Could you check a few things on this model? Use its own coordinates, in mm. Face numbers are marked on the shaded views. A direction names the side the tool comes from. Give positions to 0.01 mm unless a question says otherwise; leave off trailing zeros. Loops run counter-clockwise (first coordinate to the right, second up) from the corner with the lowest first, then second, coordinate; pieces in that order, holes last. Notation, with made-up numbers: M 28.25,60.5 L 63.25,60.5 A28 ccw 63.25,78.5 Z; hole C 39.25,-36 d9. An arc over 180 degrees is marked long. Answer in a Markdown table with one row per item. Add a question column.
1. Which directions (+Z, -Z, +X, -X, +Y, -Y) give clear straight access to the entire face, cutting with the end or side of a thin tool? Please do the marked faces 1 and 2.
2. If we section it at A-A on x = 12: List the corners of the cut face in (y, z) for me, then the cut area to 3 significant figures.
3. Thinking about a two-plate mould opening in Y: for the marked faces 3, 4 and 5, which applies, released by +Y, released by -Y, zero draft, split by the parting line, or undercut?
4. If we section it at B-B on z = 2.8: List the corners of the cut face in (x, y) for me.
5. If we section it at D-D on z = 1.05: List the corners of the cut face in (x, y) for me, then the cut area to 3 significant figures.
6. If we section it at C-C on y = 4.5: List the corners of the cut face in (x, z) for me.
7. I need wall thicknesses on line 1 along Y through (x, z) = (14.5, 2.5); line 2 along Y through (x, z) = (-10.5, 0.2); line 3 along Z through (x, y) = (5, 1.75). Which ranges of each line are inside material? Lowest first, please. Write a range as from..to.
8. I'm going to push flat-ended pins straight in: pin 1 Ø0.9 at (x, z) = (7.5, 4) entering from +Y; pin 2 Ø1.5 at (x, z) = (12.5, 4) entering from -Y; pin 3 Ø2 at (y, z) = (3, 4) entering from -X; pin 4 Ø2.5 at (x, z) = (11, 2.5) entering from +Y. Where does each tip first touch, or does it pass through?
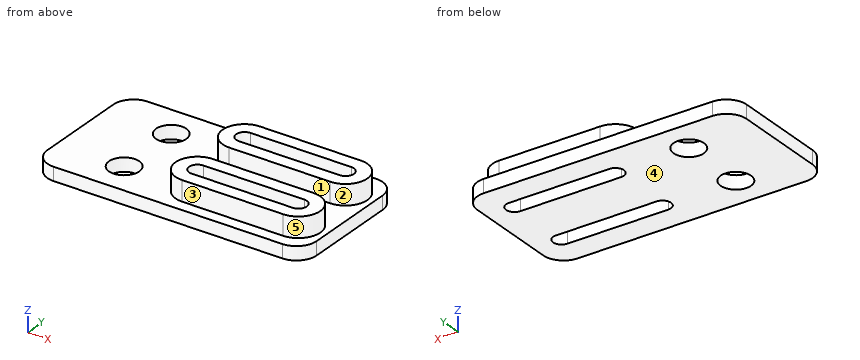
```python
from build123d import *

# Parameters (mm, degrees)
SZKIC1_W                    = 40
SZKIC1_H                    = 20
SZKIC1_R                    = 2.25
DODANIE_WYCI_GNI_CIE1_DEPTH = 2
DODANIE_WYCI_GNI_CIE2_DEPTH = 5
ZAOKR_GLENIE1_R             = 3


with BuildPart() as part:
    # Szkic1 → Dodanie-wyci_gni_cie1 (new body)
    with BuildSketch(Plane.XY):
        with Locations((0.494567618, 0.286392586)):
            Rectangle(SZKIC1_W, SZKIC1_H)
        with Locations((-9.505432382, -4.713607414)):
            Circle(SZKIC1_R, mode=Mode.SUBTRACT)
        with Locations((-9.505432382, 5.286392586)):
            Circle(SZKIC1_R, mode=Mode.SUBTRACT)
        with BuildLine():
            ThreePointArc((16.387577827, 2.036392586), (19.637577827, 5.286392586), (16.387577827, 8.536392586))
            Line((16.387577827, 8.536392586), (1.387577827, 8.536392586))
            ThreePointArc((1.387577827, 8.536392586), (-1.862422173, 5.286392586), (1.387577827, 2.036392586))
            Line((1.387577827, 2.036392586), (16.387577827, 2.036392586))
        make_face(mode=Mode.SUBTRACT)
        with BuildLine():
            ThreePointArc((16.387577827, -7.963607414), (19.637577827, -4.713607414), (16.387577827, -1.463607414))
            Line((16.387577827, -1.463607414), (1.387577827, -1.463607414))
            ThreePointArc((1.387577827, -1.463607414), (-1.862422173, -4.713607414), (1.387577827, -7.963607414))
            Line((1.387577827, -7.963607414), (16.387577827, -7.963607414))
        make_face(mode=Mode.SUBTRACT)
    extrude(amount=DODANIE_WYCI_GNI_CIE1_DEPTH)

    # Szkic1_3 → Dodanie-wyci_gni_cie2 (add)
    # profile 1 of 2: a face of its own
    with BuildSketch(Plane.XY):
        with BuildLine():
            Line((1.387577827, -1.463607414), (16.387577827, -1.463607414))
            ThreePointArc((16.387577827, -1.463607414), (19.637577827, -4.713607414), (16.387577827, -7.963607414))
            Line((16.387577827, -7.963607414), (1.387577827, -7.963607414))
            ThreePointArc((1.387577827, -7.963607414), (-1.862422173, -4.713607414), (1.387577827, -1.463607414))
        make_face()
        with BuildLine():
            Line((1.387577827, -3.463607414), (16.387577827, -3.463607414))
            ThreePointArc((16.387577827, -3.463607414), (17.637577827, -4.713607414), (16.387577827, -5.963607414))
            Line((16.387577827, -5.963607414), (1.387577827, -5.963607414))
            ThreePointArc((1.387577827, -5.963607414), (0.137577827, -4.713607414), (1.387577827, -3.463607414))
        make_face(mode=Mode.SUBTRACT)
    # profile 2 of 2: a face of its own
    with BuildSketch(Plane.XY):
        with BuildLine():
            Line((1.387577827, 8.536392586), (16.387577827, 8.536392586))
            ThreePointArc((16.387577827, 8.536392586), (19.637577827, 5.286392586), (16.387577827, 2.036392586))
            Line((16.387577827, 2.036392586), (1.387577827, 2.036392586))
            ThreePointArc((1.387577827, 2.036392586), (-1.862422173, 5.286392586), (1.387577827, 8.536392586))
        make_face()
        with BuildLine():
            Line((1.387577827, 6.536392586), (16.387577827, 6.536392586))
            ThreePointArc((16.387577827, 6.536392586), (17.637577827, 5.286392586), (16.387577827, 4.036392586))
            Line((16.387577827, 4.036392586), (1.387577827, 4.036392586))
            ThreePointArc((1.387577827, 4.036392586), (0.137577827, 5.286392586), (1.387577827, 6.536392586))
        make_face(mode=Mode.SUBTRACT)
    extrude(amount=DODANIE_WYCI_GNI_CIE2_DEPTH)

    # Zaokr_glenie1
    zaokr_glenie1_edges = [part.edges().sort_by_distance(p)[0] for p in [
        (20.494567618, -9.713607414, 1),
        (-19.505432382, -9.713607414, 1),
        (-19.505432382, 10.286392586, 1),
        (20.494567618, 10.286392586, 1),
    ]]
    fillet(zaokr_glenie1_edges, radius=ZAOKR_GLENIE1_R)


solid = part.part
```
Results:
| question | item | result |
|---|---|---|
| 1 | face 1 | +Z, +X, -X |
| 1 | face 2 | +Z, +X |
| 2 | outline | M -9.71,0 L -5.96,0 L -5.96,5 L -7.96,5 L -7.96,2 L -9.71,2 Z; M -3.46,0 L 4.04,0 L 4.04,5 L 2.04,5 L 2.04,2 L -1.46,2 L -1.46,5 L -3.46,5 Z; M 6.54,0 L 10.29,0 L 10.29,2 L 8.54,2 L 8.54,5 L 6.54,5 Z |
| 2 | area | 54.0 mm2 |
| 3 | face 3 | released by -Y |
| 3 | face 4 | zero draft |
| 3 | face 5 | undercut |
| 4 | outline | M 1.39,-7.96 L 16.39,-7.96 A3.25 ccw 16.39,-1.46 L 1.39,-1.46 A3.25 ccw Z; M 1.39,2.04 L 16.39,2.04 A3.25 ccw 16.39,8.54 L 1.39,8.54 A3.25 ccw Z; hole M 1.39,-5.96 L 16.39,-5.96 A1.25 ccw 16.39,-3.46 L 1.39,-3.46 A1.25 ccw Z; hole M 1.39,4.04 L 16.39,4.04 A1.25 ccw 16.39,6.54 L 1.39,6.54 A1.25 ccw Z |
| 5 | outline | M -19.51,-6.71 A3 ccw -16.51,-9.71 L 17.49,-9.71 A3 ccw 20.49,-6.71 L 20.49,7.29 A3 ccw 17.49,10.29 L -16.51,10.29 A3 ccw -19.51,7.29 Z; hole C -9.51,-4.71 d4.5; hole C -9.51,5.29 d4.5; hole M 1.39,-5.96 L 16.39,-5.96 A1.25 ccw 16.39,-3.46 L 1.39,-3.46 A1.25 ccw Z; hole M 1.39,4.04 L 16.39,4.04 A1.25 ccw 16.39,6.54 L 1.39,6.54 A1.25 ccw Z |
| 5 | area | 676 mm2 |
| 6 | outline | M -19.51,0 L -11.61,0 L -11.61,2 L -19.51,2 Z; M -7.4,0 L 0.42,0 L 0.42,5 L -1.77,5 L -1.77,2 L -7.4,2 Z; M 17.36,0 L 20.49,0 L 20.49,2 L 19.54,2 L 19.54,5 L 17.36,5 Z |
| 7 | line 1 | -7.96..-5.96, -3.46..-1.46, 2.04..4.04, 6.54..8.54 |
| 7 | line 2 | -9.71..-6.73, -2.7..3.27, 7.3..10.29 |
| 7 | line 3 | 0..2 |
| 8 | pin 1 | y = 8.54 |
| 8 | pin 2 | y = -7.96 |
| 8 | pin 3 | x = -1.6 |
| 8 | pin 4 | y = 10.29 |
